Can you work these out from the drawing? Everything is in mm from the part's minimum corner. Give positions to 0.01 mm unless a question says otherwise; leave off trailing zeros. Write each loop counter-clockwise with the first axis right and the second up, starting at its lowest first coordinate (ties: lowest second). Pieces come first, ordered by that corner, then holes. Notation, with made-up numbers: (-0.75, 28) - (52.25, 28) arc R22 ccw to (52.25, 52) - close; hole circle Ø10 at (-31.5, 51.5). An arc over 180 degrees is marked (long way). Write each question's results on one line, items separated by ' | '. Start each with the question number.
Item 1: Suppose I cut it at B-B on z = 3. List the corners of the cut face in (x, y) for me, then the cut area to 3 significant figures.
Item 2: Please list where these lines run through material, in increasing order: line 1 along Y through (x, z) = (2.5, 2); line 2 along X through (y, z) = (9.25, 3); line 3 along Z through (x, y) = (1.25, 5).
Item 3: We'd pull the mould along Z, two halves only. Please class the marked faces 1, 2 and 3: +Z half, -Z half, draft (parallel to the pull), parting line (faces both ways), or undercut.
Item 4: Will these pins go through, and if not, where does the flat tip stop? P1, Ø1, axis at x = 1, y = 7, coming from the +Z side; P2, Ø1, axis at x = 5.5, z = 5.5, coming from the -Y side.
Item 5: Suppose I cut it at C-C on y = 10.25. List the corners of the cut face in (x, z) for me.
Item 6: Suppose I cut it at A-A on x = 2.25. List the corners of the cut face in (y, z) for me, then the cut area to 3 significant figures.
Item 7: Suppose I cut it at D-D on x = 3. List the corners of the cut face in (y, z) for me.
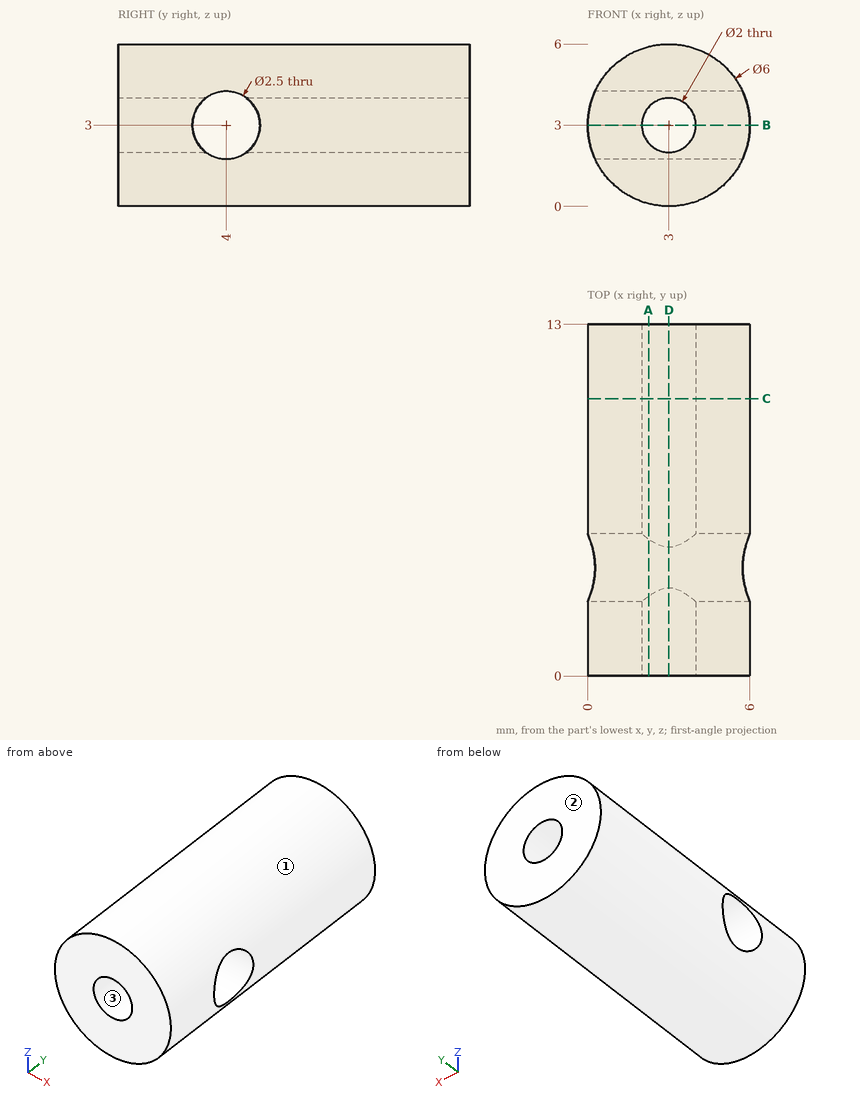
Checked values:
1) outline: (0, 0) - (2, 0) - (2, 2.75) - (0, 2.75) - close; (0, 5.25) - (2, 5.25) - (2, 13) - (0, 13) - close; (4, 0) - (6, 0) - (6, 2.75) - (4, 2.75) - close; (4, 5.25) - (6, 5.25) - (6, 13) - (4, 13) - close | area: 42.0 mm^2
2) line 1: y = 0 to 3.25, 4.75 to 13 | line 2: x = 0 to 2, 4 to 6 | line 3: z = 0.56 to 2.25, 3.75 to 5.44
3) face 1: parting line | face 2: draft | face 3: undercut
4) P1: stops at z = 5.6 | P2: passes through
5) outline: circle Ø6 at (3, 3); hole circle Ø2 at (3, 3)
6) outline: (0, 0.1) - (13, 0.1) - (13, 2.34) - (5.06, 2.34) arc R1.25 cw to (2.94, 2.34) - (0, 2.34) - close; (0, 3.66) - (2.94, 3.66) arc R1.25 cw to (5.06, 3.66) - (13, 3.66) - (13, 5.9) - (0, 5.9) - close | area: 56.6 mm^2
7) outline: (0, 0) - (13, 0) - (13, 2) - (4.75, 2) arc R1.25 cw to (3.25, 2) - (0, 2) - close; (0, 4) - (3.25, 4) arc R1.25 cw to (4.75, 4) - (13, 4) - (13, 6) - (0, 6) - close
